For this review, take the finished solid that the model builds, in its own axes (mm). Face numbers are marked on the shaded views. Give positions to 0.01 mm unless a question says otherwise; leave off trailing zeros. Write each loop counter-clockwise with the first axis right and the second up, starting at its lowest first coordinate (ties: lowest second). Pieces come first, ordered by that corner, then holes. Notation, with made-up numbers: (70, 64) -> (115, 64) arc R38 ccw to (115, 103) -> close; hole circle Ø5 at (-13.5, 64.25). An arc over 180 degrees is marked (long way). Write item = value, one per line.
```python
from build123d import *

# Parameters (mm, degrees)
SKETCH1_W                                       = 44.45
SKETCH1_H                                       = 29.972
EXTRUDE1_DEPTH                                  = 4.7625
F_10_32_TAPPED_HOLE1_D                          = 4.0386
CSK_FOR_M4_FLAT_HEAD_MACHINE_SCREW1_D           = 4.5
CSK_FOR_M4_FLAT_HEAD_MACHINE_SCREW1_CSINK_D     = 9.4
CSK_FOR_M4_FLAT_HEAD_MACHINE_SCREW1_CSINK_ANGLE = 90


with BuildPart() as part:
    # Sketch1 → Extrude1 (new body)
    with BuildSketch(Plane(origin=(0, 0, 0), x_dir=(1, 0, 0), z_dir=(0, 1, 0))):
        with Locations((22.225, 14.986)):
            Rectangle(SKETCH1_W, SKETCH1_H)
    extrude(amount=EXTRUDE1_DEPTH)

    # #10-32 Tapped Hole1 (through all)
    with Locations(Plane(origin=(0, 4.7625, 0), x_dir=(-1, 0, 0), z_dir=(0, 1, 0))):
        with Locations((-4.7625, -14.986), (-39.6875, -14.986)):
            Hole(F_10_32_TAPPED_HOLE1_D / 2)

    # CSK for M4 Flat Head Machine Screw1 (through all)
    with Locations(Plane(origin=(0, 4.7625, 0), x_dir=(-1, 0, 0), z_dir=(0, 1, 0))):
        with Locations((-28.2575, -12.7), (-16.1925, -25.4)):
            CounterSinkHole(CSK_FOR_M4_FLAT_HEAD_MACHINE_SCREW1_D / 2, CSK_FOR_M4_FLAT_HEAD_MACHINE_SCREW1_CSINK_D / 2, counter_sink_angle=CSK_FOR_M4_FLAT_HEAD_MACHINE_SCREW1_CSINK_ANGLE)


solid = part.part
```
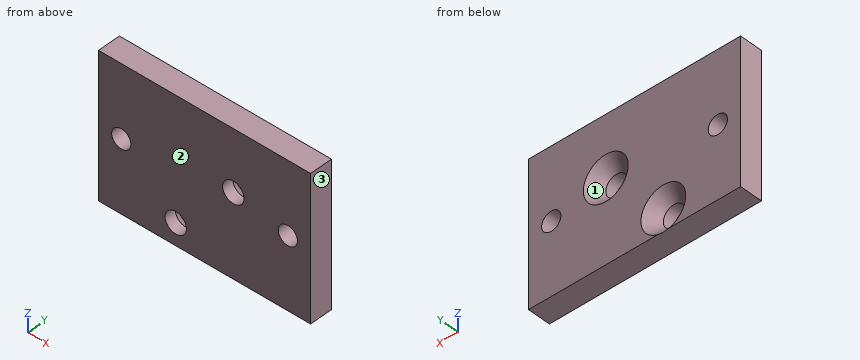
(1) The part is to be moulded in two halves that separate along X. For the marked faces 1, 2 and 3, say which applies: released by +X, released by -X, zero draft, split by the parting line, or undercut.
Answers below:
face_1 = undercut
face_2 = zero draft
face_3 = released by +X
(2) For pin 1 (2 mm diameter, centred on x = 26, z = -15.5, fed in from +Y); pin 2 (6 mm diameter, centred on x = 16.19, z = -25.4, fed in from +Y) (3 decimals); pin 3 (3.5 mm diameter, centred on x = 39.69, z = -14.99, fed in from -Y), all flat-tipped, find the tip position at first contact; note any pin that passes through.
Answers below:
pin_1 = 4.66
pin_2 = 3.065
pin_3 = through
(3) To check wall thickness, follow probe 1 along X at (y, z) = (0.75, -12.7); probe 2 along X at (y, z) = (4.25, -14.75); probe 3 along X at (y, z) = (1.2, -25.4). State the ranges of each line that lie inside material, in increasing order.
Answers below:
probe_1 = 0 to 26.01, 30.51 to 44.45
probe_2 = 0 to 2.76, 6.77 to 24.61, 31.91 to 37.68, 41.69 to 44.45
probe_3 = 0 to 13.94, 18.44 to 44.45
(4) Take a section at A-A (z = -25.4). Write out the cut boundary in (x, y), plus the area to 3 significant figures.
Answers below:
outline = (0, 0) -> (13.94, 0) -> (13.94, 2.31) -> (11.49, 4.76) -> (0, 4.76) -> close; (18.44, 0) -> (44.45, 0) -> (44.45, 4.76) -> (20.89, 4.76) -> (18.44, 2.31) -> close
area = 184 mm^2
